Verification items for this drawing (mm, ordinates from the low corner). A direction names the side the tool comes from. Give positions to 0.01 mm unless a question says otherwise; leave off trailing zeros. Order: outer loops, then holes, each group sorted by start corner. A loop starts at its lowest first (then second) coordinate and runs counter-clockwise, first axis right, second up.
(1) Gauge pin test, flat ends, axial feed: pin 1 (6 mm diameter, centred on x = 10.5, y = 2.5, fed in from -Z); pin 2 (6 mm diameter, centred on x = 44.5, z = 38, fed in from -Y); pin 3 (6 mm diameter, centred on y = 1.5, z = 10.5, fed in from -X). Record the tip position at first contact, or that the pin passes through.
(2) Sectioned sample at C-C on y = 4. Record the cut outline in (x, z) (1 decimal).
(3) Sectioned sample at A-A on y = 8. Record the cut outline in (x, z) (1 decimal).
(4) Scan lines: L1, parallel to X at y = 10, z = 53 (1 decimal); L2, parallel to X at y = 6.5, z = 36 (1 decimal); L3, parallel to Z at x = 27, y = 6.5 (1 decimal). Record each from-to range of solid material in increasing order.
(5) Mould release check, pull along X, two halves, no side actions. Record for the marked faces 3, 4, 5 and 6: pulls with the +X half, pulls with the -X half, needs draft (parallel to the pull), parting line crosses it, or undercut.
(6) Access from +Z, -Z, +X, -X, +Y, -Y to the whole of each face (thin tool, end or side, straight path). Record for the marked faces 1 and 2.
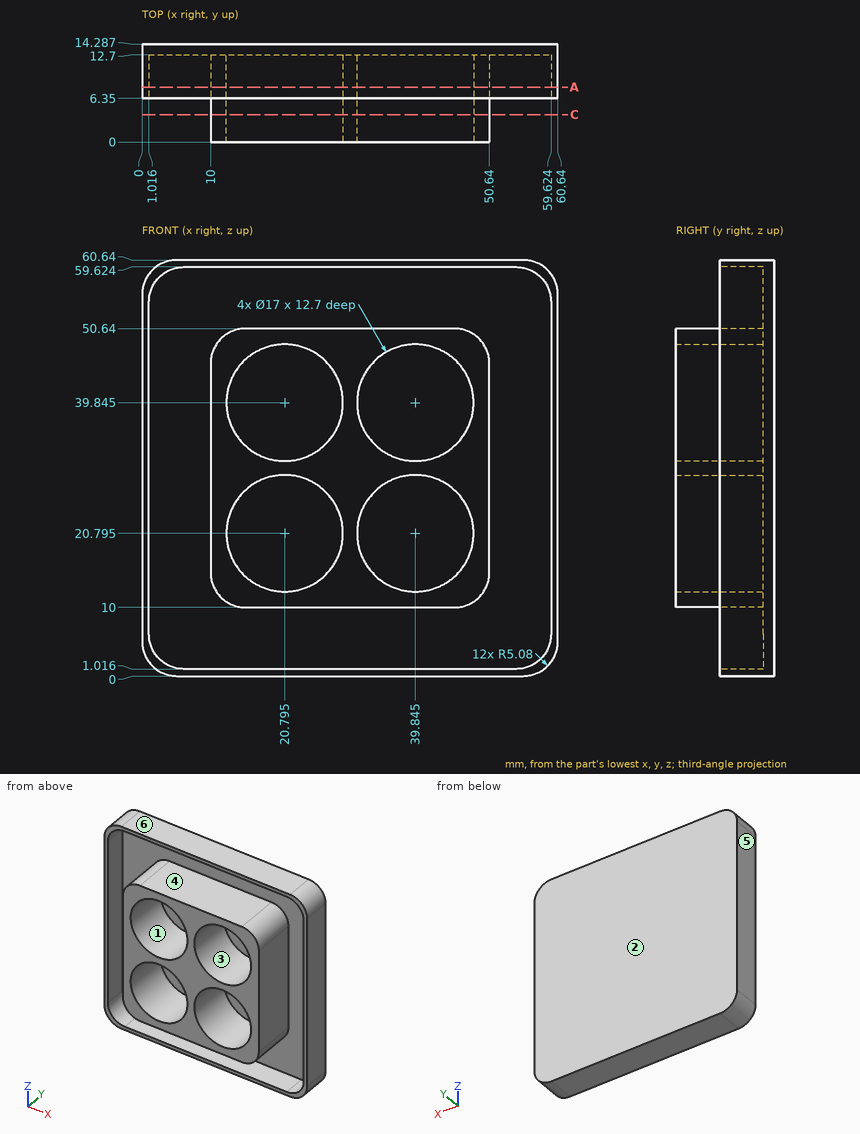
Ans:
1. pin 1: stops at z = 10.25
1. pin 2: stops at y = 12.7
1. pin 3: stops at x = 10.25
2. outline: (10, 15.1) arc R5.1 ccw to (15.1, 10) - (45.6, 10) arc R5.1 ccw to (50.6, 15.1) - (50.6, 45.6) arc R5.1 ccw to (45.6, 50.6) - (15.1, 50.6) arc R5.1 ccw to (10, 45.6) - close; hole circle Ø17 at (20.8, 20.8); hole circle Ø17 at (20.8, 39.8); hole circle Ø17 at (39.8, 20.8); hole circle Ø17 at (39.8, 39.8)
3. outline: (0, 5.1) arc R5.1 ccw to (5.1, 0) - (55.6, 0) arc R5.1 ccw to (60.6, 5.1) - (60.6, 55.6) arc R5.1 ccw to (55.6, 60.6) - (5.1, 60.6) arc R5.1 ccw to (0, 55.6) - close; (10, 15.1) arc R5.1 ccw to (15.1, 10) - (45.6, 10) arc R5.1 ccw to (50.6, 15.1) - (50.6, 45.6) arc R5.1 ccw to (45.6, 50.6) - (15.1, 50.6) arc R5.1 ccw to (10, 45.6) - close; hole (1, 6.1) arc R5.1 ccw to (6.1, 1) - (54.5, 1) arc R5.1 ccw to (59.6, 6.1) - (59.6, 54.5) arc R5.1 ccw to (54.5, 59.6) - (6.1, 59.6) arc R5.1 ccw to (1, 54.5) - close; hole circle Ø17 at (20.8, 20.8); hole circle Ø17 at (20.8, 39.8); hole circle Ø17 at (39.8, 20.8); hole circle Ø17 at (39.8, 39.8)
4. L1: x = 0 to 1, 59.6 to 60.6
4. L2: x = 0 to 1, 10 to 13.2, 28.4 to 32.3, 47.4 to 50.6, 59.6 to 60.6
4. L3: z = 0 to 1, 10 to 15, 26.6 to 34, 45.7 to 50.6, 59.6 to 60.6
5. face 3: undercut
5. face 4: undercut
5. face 5: pulls with the -X half
5. face 6: needs draft
6. face 1: -Y
6. face 2: +Z, -Z, +X, -X, +Y
